from build123d import *

# Parameters (mm, degrees)
ESQUISSE2_R             = 1.7
ENL_V_MAT_EXTRU_1_DEPTH = 10


with BuildPart() as part:
    # Esquisse1 → Révolution1 (revolve)
    with BuildSketch(Plane.XY, mode=Mode.PRIVATE) as r_volution1_sk:
        with BuildLine():
            Line((-0.5, 5), (-0.5, 10.5))
            ThreePointArc((-0.5, 10.5), (-0.353553391, 10.853553391), (0, 11))
            Line((0, 11), (2, 11))
            Line((2, 11), (2, 13.5))
            Line((2, 13.5), (1.5, 14))
            Line((1.5, 14), (0, 14))
            Line((0, 14), (0, 22.5))
            Line((0, 22.5), (-2.5, 22.5))
            Line((-2.5, 22.5), (-2.5, 5))
            Line((-2.5, 5), (-0.5, 5))
        make_face()
    revolve(r_volution1_sk.sketch.rotate(Axis((-14.777796327, 0, 0), (1, 0, 0)), 90), axis=Axis((-14.777796327, 0, 0), (1, 0, 0)))

    # Esquisse2 → Enlèv. mat.-Extru.1 (cut)
    with BuildSketch(Plane(origin=(0, 0, 0), x_dir=(0, 0, -1), z_dir=(1, 0, 0))):
        with Locations((0, 18)):
            Circle(ESQUISSE2_R)
        with Locations((15.588457268, -9)):
            Circle(ESQUISSE2_R)
        with Locations((-15.588457268, -9)):
            Circle(ESQUISSE2_R)
    extrude(amount=-ENL_V_MAT_EXTRU_1_DEPTH, mode=Mode.SUBTRACT)


solid = part.part
Geometry: final body of the model. Coordinates: model frame, mm. A direction names the side the tool comes from. Give positions to 0.01 mm unless a question says otherwise; leave off trailing zeros. Order: outer loops, then holes, each group sorted by start corner. A loop starts at its lowest first (then second) coordinate and runs counter-clockwise, first axis right, second up. Notation, with made-up numbers: (66, -32) -> (118, -32) arc R18 ccw to (118, -13) -> close; hole circle Ø5 at (4, 39.5). An arc over 180 degrees is marked (long way). Answer as a JSON object with one key per item and string values.
Q1. Section B-B (y = 18). Output: boundary loops of the cut face in (x, z).
Entries:
{"outline": "(-2.5, -13.5) -> (0, -13.5) -> (0, -1.7) -> (-2.5, -1.7) -> close; (-2.5, 1.7) -> (0, 1.7) -> (0, 13.5) -> (-2.5, 13.5) -> close"}
Q2. Section C-C (z = -16.5). Output: boundary loops of the cut face in (x, y).
Entries:
{"outline": "(-2.5, -15.3) -> (0, -15.3) -> (0, -10.43) -> (-2.5, -10.43) -> close; (-2.5, -7.57) -> (0, -7.57) -> (0, 15.3) -> (-2.5, 15.3) -> close"}
Q3. Access query for faces 5 (the cylindrical face through (1.01, 10.74, -2.38)), 6 (the cylindrical face through (-1, 0, -5)). Directions: +Z, -Z, +X, -X, +Y, -Y. A direction counts if a zero-diameter tool reaches every point of the face in a straight line with its end or side. Return the directions, or none.
Entries:
{"face 5": "+X", "face 6": "+X, -X"}
Q4. First-contact query: pin 1 (4 mm diameter, centred on y = -9, z = -14, fed in from +X); pin 2 (6.5 mm diameter, centred on y = 1.5, z = 0.5, fed in from +X); pin 3 (1.5 mm diameter, centred on x = -0.5, z = -1, fed in from +Y); pin 4 (1.5 mm diameter, centred on x = -1, y = 14, fed in from +Z). Flat tips, straight axial feed; report the tip coordinate or a pass-through.
Entries:
{"pin 1": "stops at x = 0", "pin 2": "passes through", "pin 3": "stops at y = 22.5", "pin 4": "stops at z = 18.18"}
Q5. Section A-A (z = 0). Output: boundary loops of the cut face in (x, y).
Entries:
{"outline": "(-2.5, -22.5) -> (0, -22.5) -> (0, -14) -> (1.5, -14) -> (2, -13.5) -> (2, -11) -> (0, -11) arc R0.5 cw to (-0.5, -10.5) -> (-0.5, -5) -> (-2.5, -5) -> close; (-2.5, 5) -> (-0.5, 5) -> (-0.5, 10.5) arc R0.5 cw to (0, 11) -> (2, 11) -> (2, 13.5) -> (1.5, 14) -> (0, 14) -> (0, 16.3) -> (-2.5, 16.3) -> close; (-2.5, 19.7) -> (0, 19.7) -> (0, 22.5) -> (-2.5, 22.5) -> close"}
Q6. Section D-D (x = 0.8). Output: boundary loops of the cut face in (y, z), plus the area to 3 significant figures.
Entries:
{"outline": "circle Ø28 at (0, 0); hole circle Ø22 at (0, 0)", "area": "236 mm^2"}
Q7. Material intervals for probe 1 along Y at (x, z) = (-0.9, 0); probe 2 along X at (y, z) = (-13, 13.5); probe 3 along Y at (x, z) = (1.2, 0), sorted ascending.
Entries:
{"probe 1": "y = -22.5 to -5, 5 to 16.3, 19.7 to 22.5", "probe 2": "x = -2.5 to 0", "probe 3": "y = -14 to -11, 11 to 14"}
Q8. Draft query along Y for faces 1 (the cylindrical face through (-1.268, 19.961, 10.382)), 2 (the flat face through (0, 15, 0)), 3 (the cylindrical face through (-1.23, -8.93, -13.89)), 4 (the flat face through (-0.5, 2, -5)). Return one class per face: released by +Y, released by -Y, zero draft, split by the parting line, or undercut.
Entries:
{"face 1": "split by the parting line", "face 2": "zero draft", "face 3": "undercut", "face 4": "undercut"}
